Could you check a few things on this drawing? It's one solid part, dimensions in mm from its lowest x, y, z. Round coordinates to 2 decimals unless told otherwise and drop trailing zeros. Write each loop counter-clockwise with the first axis right and the second up, starting at its lowest first coordinate (ties: lowest second). Pieces come first, ordered by that corner, then holes. Notation, with made-up numbers: (53, 77.25) -> (96, 77.25) arc R20 cw to (96, 81.25) -> close; hole circle Ø6 at (22.25, 47). An arc over 180 degrees is marked (long way). Put each result on its own line as item: value. Start each with the question number.
1) I want a section at D-D, the plane x = 10. List the corners of the cut face in (y, z) for me.
2) Will this pin go through, and if not, where does the flat tip stop? P1, Ø1.3, axis at x = 4, z = 4, coming from the -Y side.
3) I want a section at B-B, the plane y = 0.7. List the corners of the cut face in (x, z) for me.
4) If I drill on line 1 along X through (y, z) = (1.7, 28.8); line 2 along X through (y, z) = (1.5, 26.63); line 3 along Z through (x, y) = (7.5, 0.65), over which ranges is the centre line in solid material (lowest first)? Write a range as [from, to].
5) I want a section at A-A, the plane z = 4. List the corners of the cut face in (x, y) for me.
6) I want a section at C-C, the plane x = 16. List the corners of the cut face in (y, z) for me, then the cut area to 3 significant figures.
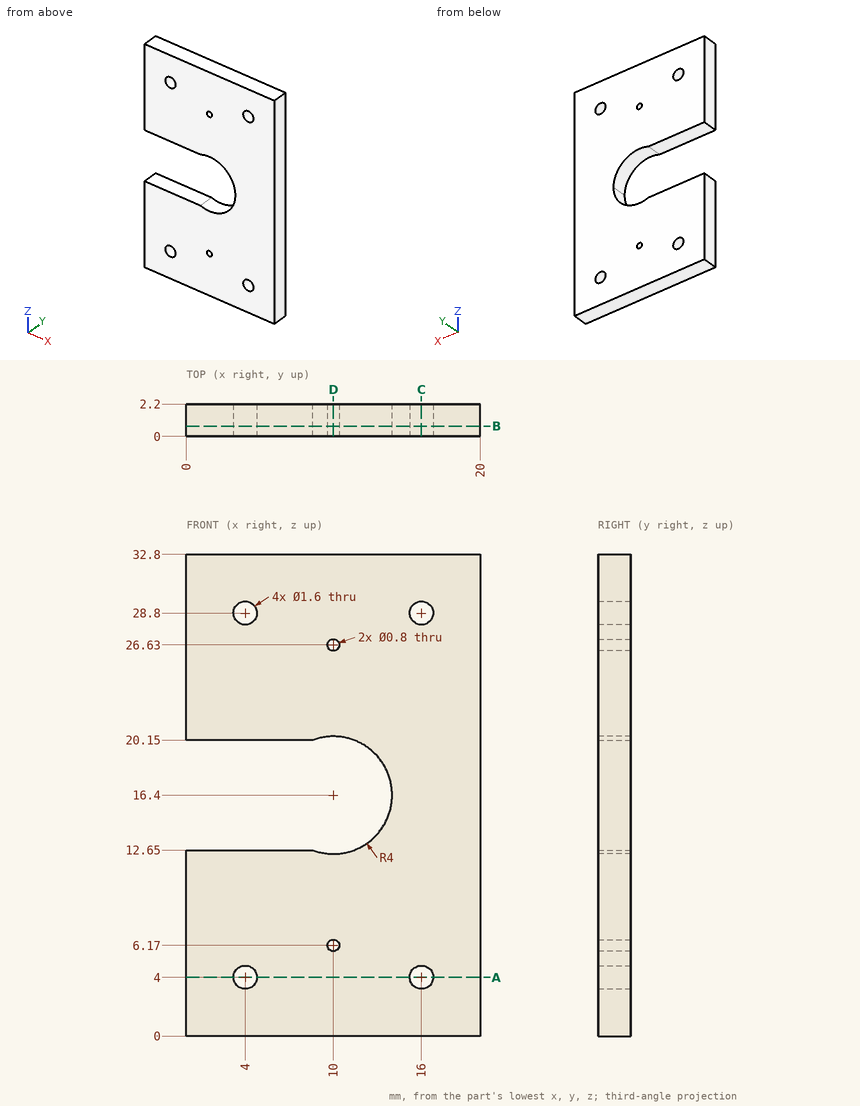
Findings:
1. outline: (0, 0) -> (2.2, 0) -> (2.2, 5.77) -> (0, 5.77) -> close; (0, 6.57) -> (2.2, 6.57) -> (2.2, 12.4) -> (0, 12.4) -> close; (0, 20.4) -> (2.2, 20.4) -> (2.2, 26.23) -> (0, 26.23) -> close; (0, 27.03) -> (2.2, 27.03) -> (2.2, 32.8) -> (0, 32.8) -> close
2. P1: passes through
3. outline: (0, 0) -> (20, 0) -> (20, 32.8) -> (0, 32.8) -> (0, 20.15) -> (8.61, 20.15) arc R4 cw (long way) to (8.61, 12.65) -> (0, 12.65) -> close; hole circle Ø1.6 at (4, 4); hole circle Ø1.6 at (4, 28.8); hole circle Ø0.8 at (10, 6.17); hole circle Ø0.8 at (10, 26.63); hole circle Ø1.6 at (16, 4); hole circle Ø1.6 at (16, 28.8)
4. line 1: x = [0, 3.2], [4.8, 15.2], [16.8, 20]
4. line 2: x = [0, 9.6], [10.4, 20]
4. line 3: z = [0, 12.65], [20.15, 32.8]
5. outline: (0, 0) -> (3.2, 0) -> (3.2, 2.2) -> (0, 2.2) -> close; (4.8, 0) -> (15.2, 0) -> (15.2, 2.2) -> (4.8, 2.2) -> close; (16.8, 0) -> (20, 0) -> (20, 2.2) -> (16.8, 2.2) -> close
6. outline: (0, 0) -> (2.2, 0) -> (2.2, 3.2) -> (0, 3.2) -> close; (0, 4.8) -> (2.2, 4.8) -> (2.2, 28) -> (0, 28) -> close; (0, 29.6) -> (2.2, 29.6) -> (2.2, 32.8) -> (0, 32.8) -> close
6. area: 65.1 mm2
